Read the model definition and answer for the solid it produces. Units are mm, in the model's axes. A direction names the side the tool comes from. Coordinates: 2 decimals unless noted, no trailing zeros. Write each loop counter-clockwise with the first axis right and the second up, starting at its lowest first coordinate (ties: lowest second). Pieces come first, ordered by that corner, then holes. Notation, with made-up numbers: (45.5, 77) -> (78.5, 77) arc R24 ccw to (78.5, 102) -> close; hole circle Ø9 at (-38, 41). An arc over 180 degrees is marked (long way). One line per item, written item: value. Start each with the question number.
1. For a pull along Z with two mould halves and no side action, classify faces 1 (the flat face through (9.3, 0, -9.3)), 2 (the flat face through (11, 5, -37)) as pulls with the +Z half, pulls with the -Z half, needs draft (parallel to the pull), parting line crosses it, or undercut.
2. Given P1, Ø1.6, axis at y = 3.5, z = 0.5, coming from the -X side; P2, Ø8, axis at x = 25.5, z = 25, coming from the +Y side; P3, Ø3, axis at x = 29, z = -21.5, coming from the -Y side, each flat-ended and moving along its own axis, determine where each tip first touches the part or whether it passes through.
3. Consider line 1 along X through (y, z) = (8.95, 0); line 2 along X through (y, z) = (4.5, 19.5); line 3 along X through (y, z) = (2.5, -8.5). Determine where each line is inside the solid, lowest interval first.
4. Find section B-B, the plane y = 11.75. State how many separate pieces and enclosed holes the cut face has, and give its area (3 significant figures).
5. For faces 3 (the flat face through (8.826, 2.465, -34.833)), 4 (the cylindrical face through (-20.462, 15.07, 29.222)), 5 (the flat face through (0, 20, -37)), determine the directions among +Z, -Z, +X, -X, +Y, -Y from which every point of the face is accessible in a straight line to the end or side of a thin tool.
6. Find section D-D, the plane x = 17.5. Write down the section's boundary in (y, z).
7. Find section A-A, the plane x = 0. Write down the section's boundary in (y, z).
```python
from build123d import *

# Parameters (mm, degrees)
CUT_EXTRUDE1_DEPTH      = 59.142067387
CUT_EXTRUDE1_DEPTH_BACK = 59.142067387
SKETCH2_R               = 1.7
SKETCH2_R_2             = 1.5
SKETCH3_W               = 7
SKETCH3_H               = 4
CUT_EXTRUDE2_DEPTH      = 5
BOSS_EXTRUDE1_START     = -20
SKETCH5_R               = 1.7
BOSS_EXTRUDE1_DEPTH     = 20


with BuildPart() as part:
    # Sketch1 → Revolve1 (revolve)
    with BuildSketch(Plane.XY, mode=Mode.PRIVATE) as revolve1_sk:
        Polygon((-29, 10), (-40.5, 10), (-40.5, 0), (-13, 0), (-13, 7.75), (-29, 7.75), align=None)
    revolve(revolve1_sk.sketch.rotate(Axis((0, -1.751877994, 0), (0, 1, 0)), 270), axis=Axis((0, -1.751877994, 0), (0, 1, 0)))

    # Sketch2 → Cut-Extrude1 (cut, two sides: drawn at the far end of the back side and taken through both)
    with BuildSketch(Plane(origin=(0, 10, 0), x_dir=(1, 0, 0), z_dir=(0, 1, 0)).offset(-CUT_EXTRUDE1_DEPTH_BACK)):
        with Locations(Location((0, 37.25, 0), (0, 0, 270))):
            Circle(SKETCH2_R)
        with Locations(Location((11.51088304, 35.426855232, 0), (0, 0, 270))):
            Circle(SKETCH2_R_2)
        with Locations(Location((21.895000648, 30.13588304, 0), (0, 0, 270))):
            Circle(SKETCH2_R)
        with Locations(Location((30.13588304, 21.895000648, 0), (0, 0, 270))):
            Circle(SKETCH2_R_2)
        with Locations(Location((35.426855232, 11.51088304, 0), (0, 0, 270))):
            Circle(SKETCH2_R)
        with Locations(Location((37.25, 0, 0), (0, 0, 270))):
            Circle(SKETCH2_R_2)
        with Locations(Location((35.426855232, -11.51088304, 0), (0, 0, 270))):
            Circle(SKETCH2_R)
        with Locations(Location((30.13588304, -21.895000648, 0), (0, 0, 270))):
            Circle(SKETCH2_R_2)
        with Locations(Location((21.895000648, -30.13588304, 0), (0, 0, 270))):
            Circle(SKETCH2_R)
        with Locations(Location((11.51088304, -35.426855232, 0), (0, 0, 270))):
            Circle(SKETCH2_R_2)
        with Locations(Location((0, -37.25, 0), (0, 0, 270))):
            Circle(SKETCH2_R)
        with Locations(Location((-11.51088304, -35.426855232, 0), (0, 0, 270))):
            Circle(SKETCH2_R_2)
        with Locations(Location((-21.895000648, -30.13588304, 0), (0, 0, 270))):
            Circle(SKETCH2_R)
        with Locations(Location((-30.13588304, -21.895000648, 0), (0, 0, 270))):
            Circle(SKETCH2_R_2)
        with Locations(Location((-35.426855232, -11.51088304, 0), (0, 0, 270))):
            Circle(SKETCH2_R)
        with Locations(Location((-37.25, 0, 0), (0, 0, 270))):
            Circle(SKETCH2_R_2)
        with Locations(Location((-35.426855232, 11.51088304, 0), (0, 0, 270))):
            Circle(SKETCH2_R)
        with Locations(Location((-30.13588304, 21.895000648, 0), (0, 0, 270))):
            Circle(SKETCH2_R_2)
        with Locations(Location((-21.895000648, 30.13588304, 0), (0, 0, 270))):
            Circle(SKETCH2_R)
        with Locations(Location((-11.51088304, 35.426855232, 0), (0, 0, 270))):
            Circle(SKETCH2_R_2)
    extrude(amount=CUT_EXTRUDE1_DEPTH + CUT_EXTRUDE1_DEPTH_BACK, mode=Mode.SUBTRACT)

    # Sketch3 → Cut-Revolve1 (revolve, cut)
    with BuildSketch(Plane.XY, mode=Mode.PRIVATE) as cut_revolve1_sk:
        with Locations((25, 2)):
            Rectangle(SKETCH3_W, SKETCH3_H)
    revolve(cut_revolve1_sk.sketch.rotate(Axis((0, -19.065406541, 0), (0, 1, 0)), 90), axis=Axis((0, -19.065406541, 0), (0, 1, 0)), mode=Mode.SUBTRACT)

    # Sketch4 → Cut-Extrude2 (cut)
    with BuildSketch(Plane.XZ):
        Polygon((10.850674752, 38.532891025), (8.490872994, 36.408115979), (9.151081283, 33.302080186), (12.171091329, 32.320819439), (14.530893087, 34.445594485), (13.870684798, 37.551630278), align=None)
        Polygon((33.293914202, 22.226923098), (31.427445347, 24.795897085), (28.269414185, 24.463974635), (26.977851878, 21.563078198), (28.844320733, 18.994104211), (32.002351895, 19.326026661), align=None)
        Polygon((40, -1.58771324), (40, 1.58771324), (37.25, 3.175426481), (34.5, 1.58771324), (34.5, -1.58771324), (37.25, -3.175426481), align=None)
        Polygon((31.427445347, -24.795897085), (33.293914202, -22.226923098), (32.002351895, -19.326026661), (28.844320733, -18.994104211), (26.977851878, -21.563078198), (28.269414185, -24.463974635), align=None)
        Polygon((10.850674752, -38.532891025), (13.870684798, -37.551630278), (14.530893087, -34.445594485), (12.171091329, -32.320819439), (9.151081283, -33.302080186), (8.490872994, -36.408115979), align=None)
        Polygon((-13.870684798, -37.551630278), (-10.850674752, -38.532891025), (-8.490872994, -36.408115979), (-9.151081283, -33.302080186), (-12.171091329, -32.320819439), (-14.530893087, -34.445594485), align=None)
        Polygon((-33.293914202, -22.226923098), (-31.427445347, -24.795897085), (-28.269414185, -24.463974635), (-26.977851878, -21.563078198), (-28.844320733, -18.994104211), (-32.002351895, -19.326026661), align=None)
        Polygon((-40, 1.58771324), (-40, -1.58771324), (-37.25, -3.175426481), (-34.5, -1.58771324), (-34.5, 1.58771324), (-37.25, 3.175426481), align=None)
        Polygon((-31.427445347, 24.795897085), (-33.293914202, 22.226923098), (-32.002351895, 19.326026661), (-28.844320733, 18.994104211), (-26.977851878, 21.563078198), (-28.269414185, 24.463974635), align=None)
        Polygon((-10.850674752, 38.532891025), (-13.870684798, 37.551630278), (-14.530893087, 34.445594485), (-12.171091329, 32.320819439), (-9.151081283, 33.302080186), (-8.490872994, 36.408115979), align=None)
    extrude(amount=-CUT_EXTRUDE2_DEPTH, mode=Mode.SUBTRACT)

    # Sketch5 → Boss-Extrude1 (add)
    with BuildSketch(Plane.XZ.offset(BOSS_EXTRUDE1_START)):
        with Locations(Location((21.895000648, 30.13588304, 0), (0, 0, 270))):
            Circle(SKETCH5_R)
        with Locations(Location((35.426855232, 11.51088304, 0), (0, 0, 270))):
            Circle(SKETCH5_R)
        with Locations(Location((35.426855232, -11.51088304, 0), (0, 0, 270))):
            Circle(SKETCH5_R)
        with Locations(Location((21.895000648, -30.13588304, 0), (0, 0, 270))):
            Circle(SKETCH5_R)
        with Locations(Location((0, -37.25, 0), (0, 0, 270))):
            Circle(SKETCH5_R)
        with Locations(Location((-35.426855232, 11.51088304, 0), (0, 0, 270))):
            Circle(SKETCH5_R)
        with Locations(Location((-21.895000648, 30.13588304, 0), (0, 0, 270))):
            Circle(SKETCH5_R)
        with Locations(Location((0, 37.25, 0), (0, 0, 270))):
            Circle(SKETCH5_R)
        with Locations(Location((-21.895000648, -30.13588304, 0), (0, 0, 270))):
            Circle(SKETCH5_R)
        with Locations(Location((-35.426855232, -11.51088304, 0), (0, 0, 270))):
            Circle(SKETCH5_R)
    extrude(amount=BOSS_EXTRUDE1_DEPTH)


solid = part.part
```
Answer block:
1. face 1: needs draft
1. face 2: undercut
2. P1: stops at x = -40.5
2. P2: stops at y = 10
2. P3: stops at y = 5
3. line 1: x = -40.5 to -38.75, -35.75 to -29, 29 to 35.75, 38.75 to 40.5
3. line 2: x = -35.5 to -32.08, -28.48 to 28.48, 32.08 to 35.5
3. line 3: x = -39.6 to -27.2, -19.75 to -9.84, 9.84 to 19.75, 27.2 to 39.6
4. separate pieces: 10
4. enclosed holes: 0
4. area: 90.8 mm2
5. face 3: -Y
5. face 4: +Y
5. face 5: +Z, -Z, +X, -X, +Y
6. outline: (0, -36.52) -> (10, -36.52) -> (10, -23.12) -> (7.75, -23.12) -> (7.75, 23.12) -> (10, 23.12) -> (10, 36.52) -> (0, 36.52) -> (0, 22.49) -> (4, 22.49) -> (4, 12.49) -> (0, 12.49) -> (0, -12.49) -> (4, -12.49) -> (4, -22.49) -> (0, -22.49) -> close
7. outline: (0, -40.5) -> (10, -40.5) -> (10, -38.95) -> (20, -38.95) -> (20, -35.55) -> (10, -35.55) -> (10, -29) -> (7.75, -29) -> (7.75, -13) -> (0, -13) -> (0, -21.5) -> (4, -21.5) -> (4, -28.5) -> (0, -28.5) -> close; (0, 13) -> (7.75, 13) -> (7.75, 29) -> (10, 29) -> (10, 35.55) -> (20, 35.55) -> (20, 38.95) -> (10, 38.95) -> (10, 40.5) -> (0, 40.5) -> (0, 28.5) -> (4, 28.5) -> (4, 21.5) -> (0, 21.5) -> close
